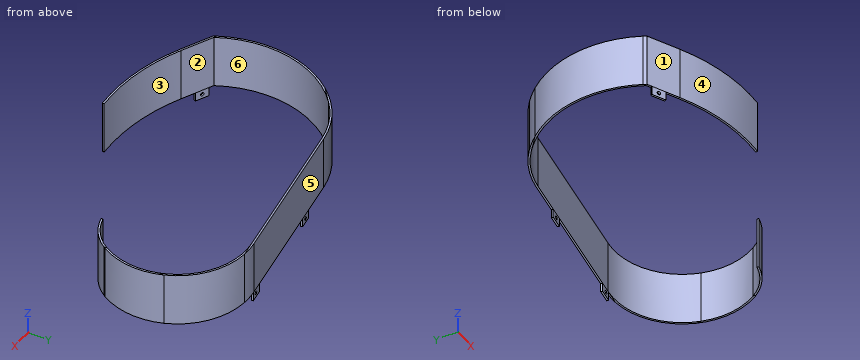
Autodesk Inventor part; units mm, degrees
ref_plane "YZ Plane" through (0, 0, 0) normal (1, 0, 0) x (0, 1, 0)
ref_plane "XZ Plane" through (0, 0, 0) normal (0, 1, 0) x (-1, 0, 0)
ref_plane "XY Plane" through (0, 0, 0) normal (0, 0, 1) x (1, 0, 0)
ref_plane "Work Plane1" through (0, 0, 0) normal (0, 0, 1) x (1, 0, 0)
sketch "Sketch1" plane through (0, 0, 0) normal (0, 0, 1) x (1, 0, 0)
  line L0 (-149.3377, -84.2183) -> (-62.5438, -127.8928)
  arc A0 (-30.3276, 119.385) -> (-94.7251, 90.539) centre (-12.6526, -6.379) ccw
  line L1 (-94.7251, 90.539) -> (-158.4791, 36.5506)
  line L2 (267.4038, 161.2284) -> (-30.3276, 119.385)
  arc A1 (285.61, 2.6867) -> (293.3792, 54.1689) centre (225.4026, 38.1) ccw
  line L3 (293.3792, 54.1689) -> (297.7515, 151.832)
  line L4 (297.7015, -118.5771) -> (285.61, 2.6867)
  line L5 (-30.3276, 119.385) -> (187.1449, 149.9488)
  arc A2 (285.61, 2.6867) -> (187.1449, 149.9488) centre (200.8332, 52.5515) ccw
  arc A3 (240.6498, -30.0656) -> (285.61, 2.6867) centre (225.4026, 38.1) ccw
  arc A4 (-30.3276, 119.385) -> (-94.7251, 90.539) centre (-12.6526, -6.379) ccw
  line L6 (-149.3377, -84.2183) -> (-62.5438, -127.8928)
  line L7 (-129.8851, -94.0069) -> (-87.7502, -115.209)
  arc A5 (-94.7251, 90.539) -> (-129.8851, -94.0069) centre (1.8279, -23.4787) ccw
  arc A6 (-87.7502, -115.209) -> (48.8152, -143.0877) centre (31.9315, 122.6334) ccw
  arc A7 (-88.9193, -117.5324) -> (48.8152, -145.6938) centre (31.9315, 122.6334) ccw
  line L8 (-88.9193, -117.5324) -> (-131.786, -95.962)
  arc A8 (-96.406, 92.5238) -> (-131.786, -95.962) centre (1.8279, -23.4787) ccw
  arc A9 (-30.6896, 121.9607) -> (-96.406, 92.5238) centre (-12.6526, -6.379) ccw
  line L9 (-30.6896, 121.9607) -> (186.7829, 152.5244)
  arc A10 (287.8519, 1.3681) -> (186.7829, 152.5244) centre (200.8332, 52.5515) ccw
  arc A11 (240.6498, -32.7284) -> (287.8519, 1.3681) centre (225.4026, 38.1) ccw
  line L10 (48.8152, -145.6938) -> (48.8152, -143.0877)
  line L11 (240.6498, -32.7284) -> (240.6498, -30.0656)
  dimension "d24" = 2.601
extrude "Extrusion1" add sketch "Sketch1" along normal blind 76.2 contours L0 A6 L10 A7 L8 A8 | L0 A8 L1 A5 | L1 A8 A9 L9 A10 L2 A0 | L2 A10 L3 A2 | L3 A10 A11 L4 A2 | L4 A11 L11 A3
ref_plane "Work Plane2" through (-66.6974, 114.2736, 0) normal (-0.1392, 0.9903, 0) x (-0.9903, -0.1392, 0)
sketch "Sketch2" plane through (-66.6974, 114.2736, 0) normal (-0.1392, 0.9903, 0) x (-0.9903, -0.1392, 0)
  circle A0 centre (-93.8772, -6.35) radius 2.4892
  circle A1 centre (-249.4522, -6.35) radius 2.4892
  line L0 (-422.3221, 0) -> (51.093, 0)
  line L1 (-36.7272, -12.7) -> (-337.3845, -12.7)
  line L2 (-36.7272, 0) -> (-256.3369, 0)
  line L3 (-102.8977, 0) -> (-102.8977, -12.7)
  line L4 (-83.8477, -12.7) -> (-102.8977, -12.7)
  line L5 (-83.8477, -12.7) -> (-83.8477, 0)
  circle A2 centre (-93.8772, -6.35) radius 2.4892
  line L6 (-16.5377, -12.7) -> (-16.5377, 0)
  circle A3 centre (-249.4522, -6.35) radius 2.4892
  line L7 (-354.6914, 0) -> (-256.3369, 0)
  line L8 (-257.8377, -12.7) -> (-238.7877, -12.7)
  line L9 (-238.7877, -12.7) -> (-238.7877, 0)
  line L10 (-257.8377, -12.7) -> (-257.8377, 0)
  line L11 (-238.7877, 0) -> (-257.8377, 0)
  line L12 (-83.8477, 0) -> (-102.8977, 0)
  line L13 (-97.2698, 0) -> (-97.2698, 76.2)
  point P0 (-50.1445, 0)
  point P1 (-333.3488, 0)
  dimension "d7" = 19.05
  dimension "d8" = 67.31
  dimension "d9" = 135.89
  dimension "d10" = 19.05
extrude "Extrusion2" add sketch "Sketch2" along normal blind 2.601 contours L0 L9 L1 L10 | L0 L5 L1 L3
ref_plane "Work Plane5" through (6.35, -162.56, 0) normal (-0.4495, -0.8933, 0) x (0.8933, -0.4495, 0)
sketch "Sketch5" plane through (6.35, -162.56, 0) normal (-0.4495, -0.8933, 0) x (0.8933, -0.4495, 0)
  circle A0 centre (-135.8153, -6.35) radius 2.4892
  line L0 (-174.2873, 0) -> (-77.1244, 0)
  line L1 (-77.1244, -12.7) -> (-174.2873, -12.7)
  line L2 (-105.3421, 0) -> (-152.5108, 0)
  line L3 (-145.8483, 0) -> (-125.7823, 0)
  line L4 (-125.7823, 0) -> (-125.7823, -12.7)
  circle A1 centre (-135.8153, -6.35) radius 2.4892
  line L5 (-145.8483, 0) -> (-145.8483, -12.7)
  line L6 (-125.7823, -12.7) -> (-145.8483, -12.7)
  point P0 (-78.7426, 0)
  point P1 (-125.7823, 0)
  dimension "d25" = 10.033
  dimension "d26" = 10.033
extrude "Extrusion5" add sketch "Sketch5" along normal blind 2.601
properties part number "ChainGuard"
CAD build for the part. Positions are in the model's coordinates, mm. Face numbers are marked on the shaded views. A direction names the side the tool comes from. Round coordinates to 2 decimals unless told otherwise and drop trailing zeros. Write each loop counter-clockwise with the first axis right and the second up, starting at its lowest first coordinate (ties: lowest second). Pieces come first, ordered by that corner, then holes.
Item 1: Tool access for the marked faces 1, 2 and 3: list every direction of +Z, -Z, +X, -X, +Y, -Y with a clear straight run to the whole face (end or side of a thin tool).
Filled in:
face 1: +Z, -Z, -X, -Y
face 2: +Z, -Z, +X
face 3: +Z, -Z
Item 2: Mould opens along Y. For the marked faces 4, 5 and 6 say: released by +Y, released by -Y, zero draft, split by the parting line, or undercut.
Filled in:
face 4: released by -Y
face 5: released by +Y
face 6: undercut
Item 3: Band-saw the part on D-D on y = -59.5. Write the cut outline in (x, z).
Filled in:
outline: (-145.85, 0) - (-143.17, 0) - (-143.17, 76.2) - (-145.85, 76.2) - close
Item 4: Band-saw the part on A-A on x = 262.5. Write the cut outline in (y, z).
Filled in:
outline: (-24.13, 0) - (-21.08, 0) - (-21.08, 76.2) - (-24.13, 76.2) - close; (129.17, 0) - (132.48, 0) - (132.48, 76.2) - (129.17, 76.2) - close
Item 5: Drill centre lines: L1, parallel to X at y = 69, z = 19; L2, parallel to Y at x = -2.5, z = 64; L3, parallel to Y at x = -70, z = 26. Where is each one in solid material? Low to high.
Filled in:
L1: x = -118.81 to -115.52, 297.8 to 300.44
L2: y = -144.01 to -141.39, 123.3 to 125.92
L3: y = -126.15 to -123.34, 106.94 to 109.84
Item 6: Band-saw the part on B-B on y = 67.5. Write the cut outline in (x, z), then the cut area to 3 significant figures.
Filled in:
outline: (-119.95, 0) - (-116.69, 0) - (-116.69, 76.2) - (-119.95, 76.2) - close; (298.05, 0) - (300.68, 0) - (300.68, 76.2) - (298.05, 76.2) - close
area: 449 mm2
Item 7: Band-saw the part on C-C on z = 48. Write the cut outline in (x, y) (1 decimal), then the cut area to 3 significant figures.
Filled in:
outline: (-131.8, -96) - (-88.9, -117.5) arc R268.9 ccw to (48.8, -145.7) - (48.8, -143.1) arc R266.3 cw to (-87.8, -115.2) - (-129.9, -94) arc R149.4 cw to (-94.7, 90.5) arc R127 cw to (-30.3, 119.4) - (187.1, 149.9) arc R98.4 cw to (285.6, 2.7) arc R69.9 cw to (240.6, -30.1) - (240.6, -32.7) arc R72.5 ccw to (287.9, 1.4) arc R101 ccw to (186.8, 152.5) - (-30.7, 122) arc R129.6 ccw to (-96.4, 92.5) arc R152 ccw to start
area: 2,520 mm2
Item 8: Drop flat-ended pins along their axis: pin 1 Ø2 at (y, z) = (-12, 10.5) entering from -X; pin 2 Ø3 at (x, y) = (26.5, 130.5) entering from +Z; pin 3 Ø1.3 at (y, z) = (-144.5, 46.5) entering from +X; pin 4 Ø0.8 at (y, z) = (-32, 19) entering from -X. Give the stop position or say it passes through.
Filled in:
pin 1: stops at x = -149.82
pin 2: stops at z = 76.2
pin 3: stops at x = 48.82
pin 4: stops at x = -149.96
